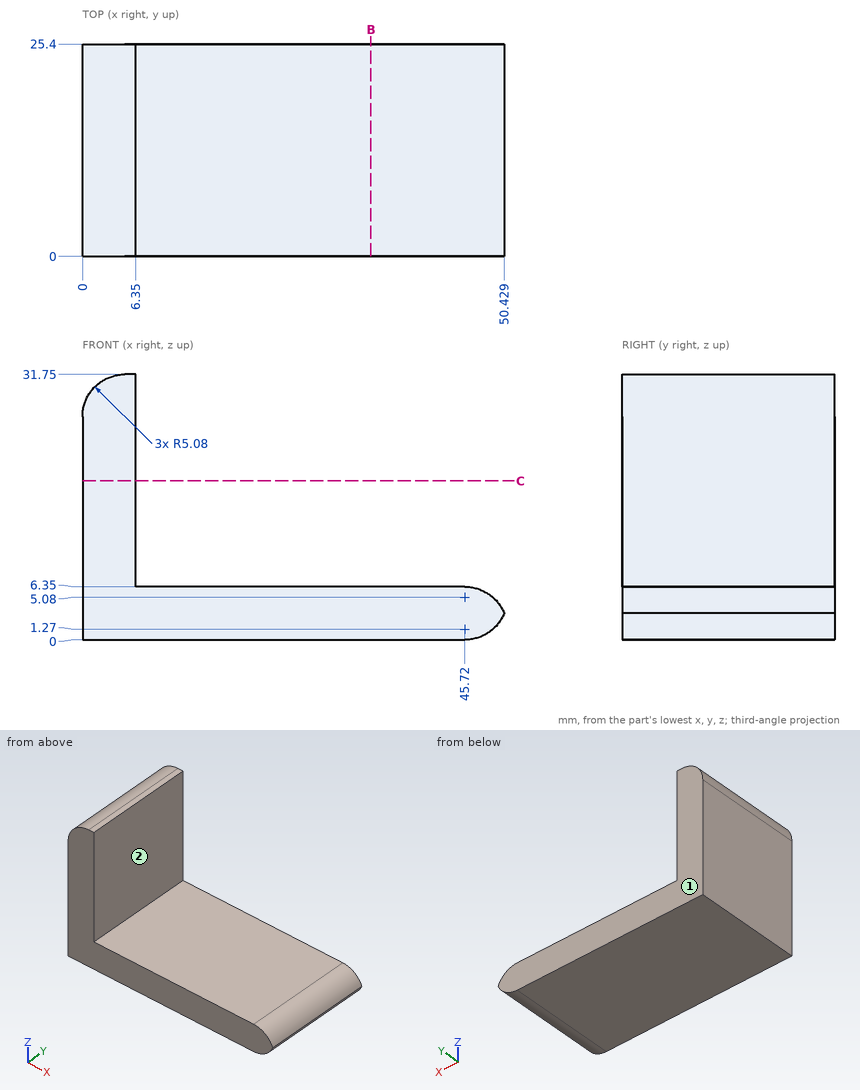
The figure shows three views and two pictorial views of one solid part (mm, origin at its lowest corner). Answer the questions. A direction names the side the tool comes from. Give positions to 0.01 mm unless a question says otherwise; leave off trailing zeros. Loops run counter-clockwise (first coordinate to the right, second up) from the corner with the lowest first, then second, coordinate; pieces in that order, holes last. Notation, with made-up numbers: (-0.75, 16) - (13.25, 16) arc R12 cw to (13.25, 36) - close; hole circle Ø11 at (-26, 61.5). An arc over 180 degrees is marked (long way). Use one line per item in the form item = value.
1. Section B-B on x = 34.5 is taken. Give the vertices of the cut face in (y, z), then the cut area to 3 significant figures.
Calculated:
outline = (0, 0) - (25.4, 0) - (25.4, 6.35) - (0, 6.35) - close
area = 161 mm^2
2. Find the intervals of material crossed by line 1 along X through (y, z) = (18.5, 27); line 2 along Z through (x, y) = (11, 10); line 3 along X through (y, z) = (6.5, 1.5) (1 decimal), in increasing order. Write a range as [from, to].
Calculated:
line_1 = [0.01, 6.35]
line_2 = [0, 6.35]
line_3 = [0, 49.3]
3. Which of the six approach directions +Z, -Z, +X, -X, +Y, -Y give full straight-line access (tool end or side, diameter ignored) to the marked faces 1 and 2?
Calculated:
face_1 = +Z, -Z, +X, -X, +Y
face_2 = +Z, +X, +Y, -Y
4. Section C-C on z = 19 is taken. Give the vertices of the cut face in (x, y).
Calculated:
outline = (0, 0) - (6.35, 0) - (6.35, 25.4) - (0, 25.4) - close
5. Given pin 1 Ø6 at (x, y) = (19.5, 18) entering from +Z; pin 2 Ø1 at (y, z) = (5, 12) entering from +X, each flat-ended and moving along its own axis, determine where each tip first touches the part or whether it passes through.
Calculated:
pin_1 = 6.35
pin_2 = 6.35
